```python
from build123d import *

# Parameters (mm, degrees)
SKETCH1_W           = 25.01
SKETCH1_H           = 33.905
BOSS_EXTRUDE1_DEPTH = 8
SKETCH2_W           = 7.55
SKETCH2_H           = 1.8
BOSS_EXTRUDE2_DEPTH = 5.495
SKETCH3_W           = 7.55
SKETCH3_H           = 1.8
BOSS_EXTRUDE3_DEPTH = 5.495
SKETCH6_R           = 1.5
CUT_EXTRUDE1_DEPTH  = 2
SKETCH8_R           = 1.5
CUT_EXTRUDE2_DEPTH  = 3
FILLET1_R           = 0.75
CHAMFER1_SIZE       = 0.5


with BuildPart() as part:
    # Sketch1 → Boss-Extrude1 (new body)
    with BuildSketch(Plane(origin=(0, 0, 0), x_dir=(1, 0, 0), z_dir=(0, 1, 0))):
        Rectangle(SKETCH1_W, SKETCH1_H)
    extrude(amount=BOSS_EXTRUDE1_DEPTH)

    # Sketch2 → Boss-Extrude2 (add)
    with BuildSketch(Plane.XY.offset(16.9525)):
        with Locations((0, 4)):
            Rectangle(SKETCH2_W, SKETCH2_H)
    extrude(amount=BOSS_EXTRUDE2_DEPTH)

    # Sketch3 → Boss-Extrude3 (add)
    with BuildSketch(Plane.ZY.offset(12.505)):
        with Locations((-13.1775, 4)):
            Rectangle(SKETCH3_W, SKETCH3_H)
    boss_extrude3 = extrude(amount=BOSS_EXTRUDE3_DEPTH)

    # Mirror2: Boss-Extrude3 across plane
    add(boss_extrude3.mirror(Plane(origin=(0, 0, 0), x_dir=(0, 0, 1), z_dir=(1, 0, 0))))

    # Sketch6 → Cut-Extrude1 (cut)
    with BuildSketch(Plane(origin=(0, 4.9, 0), x_dir=(1, 0, 0), z_dir=(0, 1, 0))):
        with Locations(Location((-15, 13.5025, 0), (0, 0, 270))):
            Circle(SKETCH6_R)
        with Locations(Location((15, 13.5025, 0), (0, 0, 270))):
            Circle(SKETCH6_R)
        with Locations(Location((0, -19.6975, 0), (0, 0, 270))):
            Circle(SKETCH6_R)
    extrude(amount=-CUT_EXTRUDE1_DEPTH, mode=Mode.SUBTRACT)

    # Sketch8 → Cut-Extrude2 (cut)
    with BuildSketch(Plane(origin=(0, 0, -16.9525), x_dir=(-1, 0, 0), z_dir=(0, 0, -1))):
        with Locations((-6.555, 4)):
            Circle(SKETCH8_R)
    extrude(amount=-CUT_EXTRUDE2_DEPTH, mode=Mode.SUBTRACT)

    # Fillet1
    fillet1_edges = [part.edges().sort_by_distance(p)[0] for p in [
        (-12.505, 8, 0),
        (12.505, 8, 0),
        (-12.505, 0, 0),
        (12.505, 0, 0),
    ]]
    fillet(fillet1_edges, radius=FILLET1_R)

    # Chamfer1
    chamfer1_edges = [part.edges().sort_by_distance(p)[0] for p in [
        (3.775, 4, 22.4475),
        (-3.775, 4, 22.4475),
        (-18, 4, -16.9525),
        (-18, 4, -9.4025),
        (18, 4, -16.9525),
        (18, 4, -9.4025),
    ]]
    chamfer(chamfer1_edges, length=CHAMFER1_SIZE)


solid = part.part
```
Source: CAD feature listing. Evaluate the final solid. Frame: model axes, mm. A direction names the side the tool comes from. Give positions to 0.01 mm unless a question says otherwise; leave off trailing zeros. Write each loop counter-clockwise with the first axis right and the second up, starting at its lowest first coordinate (ties: lowest second). Pieces come first, ordered by that corner, then holes.
1. Section query B-B (z = -4). Return the cut outline in (x, y) (3 decimals).
2. Section query A-A (x = 0). Return the cut outline in (y, z), then the cut area to 3 significant figures.
3. Access query for faces 1 (the face through (15, 4, -9.402)), 2 (the face through (16, 4.9, -12)), 3 (the face through (-16, 3.1, -12)). Directions: +Z, -Z, +X, -X, +Y, -Y. A direction counts if a zero-diameter tool reaches every point of the face in a straight line with its end or side. Return the directions, or none.
4. Material intervals for line 1 along Z through (x, y) = (-12, 0.5); line 2 along X through (y, z) = (5.75, -12) (3 decimals); line 3 along Y through (x, z) = (13.5, -11.5), sorted ascending.
5. Pull-direction query (Z, two-part tool) for faces 4 (the face through (7, 4, -13.952)), 5 (the face through (0.1, 4, 18.2)), 6 (the face through (18, 4, -13)), 7 (the face through (-14.55, 4.01, -12.07)); classes: +Z half, -Z half, draft (parallel to the pull), parting line (faces both ways), or undercut.
6. Section query D-D (x = -14.5). Return the cut outline in (y, z).
7. First-contact query: pin 1 (4 mm diameter, centred on y = 2, z = 1, fed in from -X) (3 decimals); pin 2 (4 mm diameter, centred on x = 6, y = 4.5, fed in from +Z); pin 3 (0.5 mm diameter, centred on x = 14, y = 4.5, fed in from +Z). Flat tips, straight axial feed; report the tip coordinate or a pass-through.
8. Section query C-C (y = 4). Return the cut outline in (x, z) (1 decimal).
Output values:
1. outline: (-12.505, 0.75) arc R0.75 ccw to (-11.755, 0) - (11.755, 0) arc R0.75 ccw to (12.505, 0.75) - (12.505, 7.25) arc R0.75 ccw to (11.755, 8) - (-11.755, 8) arc R0.75 ccw to (-12.505, 7.25) - close
2. outline: (0, -16.95) - (8, -16.95) - (8, 16.95) - (4.9, 16.95) - (4.9, 18.2) - (3.1, 18.2) - (3.1, 16.95) - (0, 16.95) - close; (3.1, 21.2) - (4.9, 21.2) - (4.9, 22.45) - (3.1, 22.45) - close
2. area: 276 mm2
3. face 1: +Z, +X, +Y, -Y
3. face 2: +Z, -Z, +X, +Y
3. face 3: +Z, -Z, -X, -Y
4. line 1: z = -16.95 to 16.95
4. line 2: x = -12.505 to 12.505
4. line 3: y = 3.1 to 4.9
5. face 4: -Z half
5. face 5: undercut
5. face 6: draft
5. face 7: undercut
6. outline: (3.1, -16.95) - (4.9, -16.95) - (4.9, -14.92) - (3.1, -14.92) - close; (3.1, -12.09) - (4.9, -12.09) - (4.9, -9.4) - (3.1, -9.4) - close
7. pin 1: stops at x = -12.505
7. pin 2: stops at z = 16.95
7. pin 3: stops at z = -9.4
8. outline: (-18, -16.5) - (-17.5, -17) - (5.1, -17) - (5.1, -14) - (8.1, -14) - (8.1, -17) - (17.5, -17) - (18, -16.5) - (18, -9.9) - (17.5, -9.4) - (12.5, -9.4) - (12.5, 17) - (3.8, 17) - (3.8, 21.9) - (3.3, 22.4) - (-3.3, 22.4) - (-3.8, 21.9) - (-3.8, 17) - (-12.5, 17) - (-12.5, -9.4) - (-17.5, -9.4) - (-18, -9.9) - close; hole circle Ø3 at (-15, -13.5); hole circle Ø3 at (0, 19.7); hole circle Ø3 at (15, -13.5)
